```python
from build123d import *

# Parameters (mm, degrees)
F0_W     = 4.6371185902
F0_H     = 30.6014088084
F0_H_2   = 43.4495331489
F1_DEPTH = 25.4


with BuildPart() as f1:
    # F0 (on Top) → F1 (new body)
    with BuildSketch(Plane.XY):
        with BuildLine():
            Line((63.0750581622, 37.8247536719), (-60.0328557193, 37.8247536719))
            Line((-60.0328557193, 37.8247536719), (-60.0328557193, -14.2655899338))
            Line((-60.0328557193, -14.2655899338), (-44.7080042092, 24.6659818982))
            Line((-44.7080042092, 24.6659818982), (-40.7141853078, 24.6659818982))
            Line((-40.7141853078, 24.6659818982), (-24.658497241, -16.3265038282))
            Line((-24.658497241, -16.3265038282), (-29.5725920862, -16.3265038282))
            Line((-29.5725920862, -16.3265038282), (-34.6564465714, -3.3443587191))
            Line((-34.6564465714, -3.3443587191), (-51.0159150468, -3.3443587191))
            Line((-51.0159150468, -3.3443587191), (-56.0372265067, -16.3265038282))
            Line((-56.0372265067, -16.3265038282), (-60.0328557193, -16.3265038282))
            Line((-60.0328557193, -16.3265038282), (-60.0328557193, -29.9150198698))
            Line((-60.0328557193, -29.9150198698), (6.5335062061, -29.9150198698))
            add(Edge.make_bspline(
                [(6.5335062061, -29.9150198698), (5.6202163906, -29.7963329994), (4.718855215, -29.5856251921)],
                knots=[0.5632770419, 0.5632770419, 0.5632770419, 1, 1, 1], degree=2))
            Line((4.718855215, -29.5856251921), (4.718855215, -25.8777172635))
            add(Edge.make_bspline(
                [(4.718855215, -25.8777172635), (6.2556266938, -26.2083018258), (8.1497868887, -26.2083018258)],
                knots=[0, 0, 0, 1, 1, 1], degree=2))
            add(Edge.make_bspline(
                [(8.1497868887, -26.2083018258), (12.9298609653, -26.2083018258), (14.9669766466, -20.8474710857)],
                knots=[0, 0, 0, 1, 1, 1], degree=2))
            Line((14.9669766466, -20.8474710857), (16.6735077655, -16.4962634683))
            Line((16.6735077655, -16.4962634683), (4.3257276274, 14.2749049802))
            Line((4.3257276274, 14.2749049802), (9.3023654978, 14.2749049802))
            Line((9.3023654978, 14.2749049802), (16.003403923, -3.174599079))
            add(Edge.make_bspline(
                [(16.003403923, -3.174599079), (18.2013445265, -9.1519253543), (18.7374276005, -11.8055365706)],
                knots=[0, 0, 0, 1, 1, 1], degree=2))
            Line((18.7374276005, -11.8055365706), (18.960795548, -11.8055365706))
            add(Edge.make_bspline(
                [(18.960795548, -11.8055365706), (19.318184264, -10.3759817066), (20.479697591, -6.9271805971)],
                knots=[0, 0, 0, 1, 1, 1], degree=2))
            add(Edge.make_bspline(
                [(20.479697591, -6.9271805971), (21.6412109181, -3.4783794876), (28.0652730883, 14.2749049802)],
                knots=[0, 0, 0, 1, 1, 1], degree=2))
            Line((28.0652730883, 14.2749049802), (33.0329762409, 14.2749049802))
            Line((33.0329762409, 14.2749049802), (19.8810714917, -20.5704948308))
            add(Edge.make_bspline(
                [(19.8810714917, -20.5704948308), (17.9243682716, -25.7347617771), (15.3154306447, -27.9014308679)],
                knots=[0, 0, 0, 1, 1, 1], degree=2))
            add(Edge.make_bspline(
                [(15.3154306447, -27.9014308679), (13.3999615447, -29.4921885965), (10.8439389661, -29.9150198698)],
                knots=[0, 0, 0, 0.7341950533, 0.7341950533, 0.7341950533], degree=2))
            Line((10.8439389661, -29.9150198698), (63.0750581622, -29.9150198698))
            Line((63.0750581622, -29.9150198698), (63.0750581622, 37.8247536719))
        make_face()
        with Locations((-2.9605348203, -1.025799424)):
            Rectangle(F0_W, F0_H, mode=Mode.SUBTRACT)
        with BuildLine():
            Line((60.2570616829, -16.3265038282), (56.8171952913, -16.3265038282))
            Line((56.8171952913, -16.3265038282), (55.8969193476, -11.9663614928))
            Line((55.8969193476, -11.9663614928), (55.6735514001, -11.9663614928))
            add(Edge.make_bspline(
                [(55.6735514001, -11.9663614928), (53.3862636176, -14.8433406567), (51.112377912, -15.8663658563)],
                knots=[0, 0, 0, 1, 1, 1], degree=2))
            add(Edge.make_bspline(
                [(51.112377912, -15.8663658563), (48.8384922064, -16.8893910559), (45.4254299685, -16.8893910559)],
                knots=[0, 0, 0, 1, 1, 1], degree=2))
            add(Edge.make_bspline(
                [(45.4254299685, -16.8893910559), (40.8776585573, -16.8893910559), (38.2955250841, -14.5395602481)],
                knots=[0, 0, 0, 1, 1, 1], degree=2))
            add(Edge.make_bspline(
                [(38.2955250841, -14.5395602481), (35.7133916109, -12.1897294404), (35.7133916109, -7.8653259766)],
                knots=[0, 0, 0, 1, 1, 1], degree=2))
            add(Edge.make_bspline(
                [(35.7133916109, -7.8653259766), (35.7133916109, 1.3999764859), (50.5360886075, 1.8467123809)],
                knots=[0, 0, 0, 1, 1, 1], degree=2))
            Line((50.5360886075, 1.8467123809), (55.7271597075, 2.016472021))
            Line((55.7271597075, 2.016472021), (55.7271597075, 3.9195669338))
            add(Edge.make_bspline(
                [(55.7271597075, 3.9195669338), (55.7271597075, 7.5202582476), (54.1814535108, 9.2357240844)],
                knots=[0, 0, 0, 1, 1, 1], degree=2))
            add(Edge.make_bspline(
                [(54.1814535108, 9.2357240844), (52.635747314, 10.9511899213), (49.2226850761, 10.9511899213)],
                knots=[0, 0, 0, 1, 1, 1], degree=2))
            add(Edge.make_bspline(
                [(49.2226850761, 10.9511899213), (45.3986258148, 10.9511899213), (40.5738781487, 8.6102938314)],
                knots=[0, 0, 0, 1, 1, 1], degree=2))
            Line((40.5738781487, 8.6102938314), (39.1443232846, 12.1573768378))
            add(Edge.make_bspline(
                [(39.1443232846, 12.1573768378), (41.4048069134, 13.3814331902), (44.0986243603, 14.0783411864)],
                knots=[0, 0, 0, 1, 1, 1], degree=2))
            add(Edge.make_bspline(
                [(44.0986243603, 14.0783411864), (46.7924418073, 14.7752491826), (49.5085960489, 14.7752491826)],
                knots=[0, 0, 0, 1, 1, 1], degree=2))
            add(Edge.make_bspline(
                [(49.5085960489, 14.7752491826), (54.9766434039, 14.7752491826), (57.6168525434, 12.3494732727)],
                knots=[0, 0, 0, 1, 1, 1], degree=2))
            add(Edge.make_bspline(
                [(57.6168525434, 12.3494732727), (60.2570616829, 9.9236973628), (60.2570616829, 4.5628666226)],
                knots=[0, 0, 0, 1, 1, 1], degree=2))
            Line((60.2570616829, 4.5628666226), (60.2570616829, -16.3265038282))
        make_face(mode=Mode.SUBTRACT)
        with Locations((-17.4258431008, 5.3982627463)):
            Rectangle(F0_W, F0_H_2, mode=Mode.SUBTRACT)
        with BuildLine():
            add(Edge.make_bspline(
                [(-4.8904338867, 20.2343618197), (-5.672221703, 21.0027475591), (-5.672221703, 22.5663231916)],
                knots=[0, 0, 0, 1, 1, 1], degree=2))
            add(Edge.make_bspline(
                [(-5.672221703, 22.5663231916), (-5.672221703, 24.1567029779), (-4.8904338867, 24.8982845636)],
                knots=[0, 0, 0, 1, 1, 1], degree=2))
            add(Edge.make_bspline(
                [(-4.8904338867, 24.8982845636), (-4.1086460705, 25.6398661493), (-2.9292633076, 25.6398661493)],
                knots=[0, 0, 0, 1, 1, 1], degree=2))
            add(Edge.make_bspline(
                [(-2.9292633076, 25.6398661493), (-1.8124235701, 25.6398661493), (-1.0038316001, 24.8848824867)],
                knots=[0, 0, 0, 1, 1, 1], degree=2))
            add(Edge.make_bspline(
                [(-1.0038316001, 24.8848824867), (-0.1952396302, 24.1298988242), (-0.1952396302, 22.5663231916)],
                knots=[0, 0, 0, 1, 1, 1], degree=2))
            add(Edge.make_bspline(
                [(-0.1952396302, 22.5663231916), (-0.1952396302, 21.0027475591), (-1.0038316001, 20.2343618197)],
                knots=[0, 0, 0, 1, 1, 1], degree=2))
            add(Edge.make_bspline(
                [(-1.0038316001, 20.2343618197), (-1.8124235701, 19.4659760802), (-2.9292633076, 19.4659760802)],
                knots=[0, 0, 0, 1, 1, 1], degree=2))
            add(Edge.make_bspline(
                [(-2.9292633076, 19.4659760802), (-4.1086460705, 19.4659760802), (-4.8904338867, 20.2343618197)],
                knots=[0, 0, 0, 1, 1, 1], degree=2))
        make_face(mode=Mode.SUBTRACT)
        Polygon((-44.7080042092, 24.6659818982), (-60.0328557193, -14.2655899338), (-60.0328557193, -16.3265038282), (-56.0372265067, -16.3265038282), (-51.0159150468, -3.3443587191), (-34.6564465714, -3.3443587191), (-29.5725920862, -16.3265038282), (-24.658497241, -16.3265038282), (-40.7141853078, 24.6659818982), align=None)
        with BuildLine():
            Line((-40.8839449479, 13.577996984), (-36.130675025, 0.9264364372))
            Line((-36.130675025, 0.9264364372), (-49.3361880815, 0.9264364372))
            Line((-49.3361880815, 0.9264364372), (-44.5382445691, 13.577996984))
            add(Edge.make_bspline(
                [(-42.7781051427, 19.4659760802), (-43.3946006779, 16.7855607102), (-44.5382445691, 13.577996984)],
                knots=[0, 0, 0, 1, 1, 1], degree=2))
            add(Edge.make_bspline(
                [(-40.8839449479, 13.577996984), (-41.8042208916, 15.9814360991), (-42.7781051427, 19.4659760802)],
                knots=[0, 0, 0, 1, 1, 1], degree=2))
        make_face(mode=Mode.SUBTRACT)
        Polygon((-60.0328557193, -16.3265038282), (-60.0328557193, -14.2655899338), (-60.844104737, -16.3265038282), align=None)
        with BuildLine():
            add(Edge.make_bspline(
                [(10.8439389661, -29.9150198698), (9.9185671017, -30.0680999588), (8.9092379102, -30.0680999588)],
                knots=[0.7341950533, 0.7341950533, 0.7341950533, 1, 1, 1], degree=2))
            Line((10.8439389661, -29.9150198698), (6.5335062061, -29.9150198698))
            add(Edge.make_bspline(
                [(8.9092379102, -30.0680999588), (7.7114502005, -30.0680999588), (6.5335062061, -29.9150198698)],
                knots=[0, 0, 0, 0.5632770419, 0.5632770419, 0.5632770419], degree=2))
        make_face()
        with BuildLine():
            Line((6.5335062061, -29.9150198698), (10.8439389661, -29.9150198698))
            add(Edge.make_bspline(
                [(15.3154306447, -27.9014308679), (13.3999615447, -29.4921885965), (10.8439389661, -29.9150198698)],
                knots=[0, 0, 0, 0.7341950533, 0.7341950533, 0.7341950533], degree=2))
            add(Edge.make_bspline(
                [(19.8810714917, -20.5704948308), (17.9243682716, -25.7347617771), (15.3154306447, -27.9014308679)],
                knots=[0, 0, 0, 1, 1, 1], degree=2))
            Line((19.8810714917, -20.5704948308), (33.0329762409, 14.2749049802))
            Line((33.0329762409, 14.2749049802), (28.0652730883, 14.2749049802))
            add(Edge.make_bspline(
                [(20.479697591, -6.9271805971), (21.6412109181, -3.4783794876), (28.0652730883, 14.2749049802)],
                knots=[0, 0, 0, 1, 1, 1], degree=2))
            add(Edge.make_bspline(
                [(18.960795548, -11.8055365706), (19.318184264, -10.3759817066), (20.479697591, -6.9271805971)],
                knots=[0, 0, 0, 1, 1, 1], degree=2))
            Line((18.960795548, -11.8055365706), (18.7374276005, -11.8055365706))
            add(Edge.make_bspline(
                [(16.003403923, -3.174599079), (18.2013445265, -9.1519253543), (18.7374276005, -11.8055365706)],
                knots=[0, 0, 0, 1, 1, 1], degree=2))
            Line((16.003403923, -3.174599079), (9.3023654978, 14.2749049802))
            Line((9.3023654978, 14.2749049802), (4.3257276274, 14.2749049802))
            Line((4.3257276274, 14.2749049802), (16.6735077655, -16.4962634683))
            Line((16.6735077655, -16.4962634683), (14.9669766466, -20.8474710857))
            add(Edge.make_bspline(
                [(8.1497868887, -26.2083018258), (12.9298609653, -26.2083018258), (14.9669766466, -20.8474710857)],
                knots=[0, 0, 0, 1, 1, 1], degree=2))
            add(Edge.make_bspline(
                [(4.718855215, -25.8777172635), (6.2556266938, -26.2083018258), (8.1497868887, -26.2083018258)],
                knots=[0, 0, 0, 1, 1, 1], degree=2))
            Line((4.718855215, -25.8777172635), (4.718855215, -29.5856251921))
            add(Edge.make_bspline(
                [(6.5335062061, -29.9150198698), (5.6202163906, -29.7963329994), (4.718855215, -29.5856251921)],
                knots=[0.5632770419, 0.5632770419, 0.5632770419, 1, 1, 1], degree=2))
        make_face()
    extrude(amount=F1_DEPTH)


solid = f1.part
```
Input: part model. Units: mm. Frame: model coordinates. A direction names the side the tool comes from. Coordinates: 2 decimals unless noted, no trailing zeros. Return JSON: item names as keys, results as strings.
Q1. Draft query along Y for faces 3 (the flat face through (-43, 0.926, 13)), 4 (the flat face through (-27, -29.915, 13)), 5 (the flat face through (-60.033, -23, 13)). Return one class per face: +Y half, -Y half, draft (parallel to the pull), parting line (faces both ways), or undercut.
The answers:
{"face 3": "undercut", "face 4": "-Y half", "face 5": "draft"}
Q2. First-contact query: pin 1 (6.5 mm diameter, centred on y = -10.5, z = 14, fed in from -X); pin 2 (6 mm diameter, centred on x = 46.5, z = 18, fed in from -Y) (3 decimals). Flat tips, straight axial feed; report the tip coordinate or a pass-through.
The answers:
{"pin 1": "stops at x = -60.03", "pin 2": "stops at y = -29.915"}
Q3. Ray query, probe 1 along X at (y, z) = (0, 14.5); probe 2 along X at (y, z) = (-15.5, 7.5); probe 3 along X at (y, z) = (-9.5, 17.25). Return the intervals inside material, ascending.
The answers:
{"probe 1": "x = -60.03 to -19.74, -15.11 to -5.28, -0.64 to 40.88, 60.26 to 63.08", "probe 2": "x = -60.52 to -19.74, -15.11 to -5.28, -0.64 to 39.59, 51.83 to 56.64, 60.26 to 63.08", "probe 3": "x = -60.03 to -19.74, -15.11 to -5.28, -0.64 to 35.81, 60.26 to 63.08"}
Q4. Access query for faces 1 (the flat face through (0, 4, 0)), 2 (the flat face through (-3, 14.275, 13)). Directions: +Z, -Z, +X, -X, +Y, -Y. A direction counts if a zero-diameter tool reaches every point of the face in a straight line with its end or side. Return the directions, or none.
The answers:
{"face 1": "-Z, +X, -X, +Y, -Y", "face 2": "+Z, -Z"}
Q5. Cut plane A-A (z = 12). State how many separate pieces and enclosed holes the cut face has, then the cut area to 3 significant figures.
The answers:
{"separate pieces": "1", "enclosed holes": "5", "area": "7,340 mm2"}
